The listing builds one solid part. Answer for the finished solid, in the listing's coordinates (mm). Face numbers are marked on the shaded views. Give positions to 0.01 mm unless a question says otherwise; leave off trailing zeros. Write each loop counter-clockwise with the first axis right and the second up, starting at its lowest first coordinate (ties: lowest second). Pieces come first, ordered by that corner, then holes. Notation, with made-up numbers: (36.25, 42.5) -> (94.25, 42.5) arc R21 cw to (94.25, 77.5) -> close; hole circle Ø7 at (35, -32.5). An arc over 180 degrees is marked (long way). Put each result on its own line as item: value. Start each with the question number.
1) A cutting plane is placed at D-D (z = -15). Write down the section's boundary in (x, y).
2) A cutting plane is placed at B-B (y = 3). Write down the section's boundary in (x, z), then the cut area to 3 significant figures.
3) Find the intervals of material crossed by line 1 along Z through (x, y) = (12.5, 5.5); line 2 along Y through (x, z) = (-4, -8.5); line 3 along Y through (x, z) = (0, -14), in increasing order. Write a range as from..to.
4) Flat-ended cylindrical pins translate along their axes: pin 1 Ø1.1 at (x, y) = (-21, 0.5) entering from +Z; pin 2 Ø0.5 at (x, y) = (22, 0.5) entering from -Z; pin 3 Ø4 at (x, y) = (-16, 3) entering from -Z; pin 4 Ø4 at (x, y) = (-7, 5) entering from +Z. Find the tip coordinate at first contact, or state that the pin passes through.
5) For a pull along Z with two mould halves and no side action, classify the marked faces 1, 2, 3 and 4 as released by +Z, released by -Z, zero draft, split by the parting line, or undercut.
6) A cutting plane is placed at C-C (x = -2.5). Write down the section's boundary in (y, z), then the cut area to 3 significant figures.
7) A cutting plane is placed at A-A (x = -20.5). Write down the section's boundary in (y, z), then the cut area to 3 significant figures.
from build123d import *

# Parameters (mm, degrees)
BOSS_EXTRUDE1_DEPTH   = 26.5
CUT_EXTRUDE1_DEPTH    = 2
MIRROR17_COPY_1_DEPTH = 26.5
MIRROR17_COPY_2_DEPTH = 2


with BuildPart() as part:
    # Sketch1 → Boss-Extrude1 (new body)
    with BuildSketch(Plane(origin=(0, 0, 0), x_dir=(0, 0, -1), z_dir=(1, 0, 0))):
        with BuildLine():
            Line((0, 0), (-12, 0))
            ThreePointArc((-12, 0), (-13.060660172, 0.439339828), (-13.5, 1.5))
            Line((-13.5, 1.5), (-13.5, 6))
            ThreePointArc((-13.5, 6), (-13.646446609, 6.353553391), (-14, 6.5))
            Line((-14, 6.5), (-17.5, 6.5))
            Line((-17.5, 6.5), (-17.5, 7.5))
            Line((-17.5, 7.5), (-14, 7.5))
            ThreePointArc((-14, 7.5), (-12.939339828, 7.060660172), (-12.5, 6))
            Line((-12.5, 6), (-12.5, 1.5))
            ThreePointArc((-12.5, 1.5), (-12.353553391, 1.146446609), (-12, 1))
            Line((-12, 1), (0, 1))
            Line((0, 1), (0, 0))
        make_face()
    boss_extrude1 = extrude(amount=BOSS_EXTRUDE1_DEPTH)

    # Sketch3 → Cut-Extrude1 (cut, through all)
    with BuildSketch(Plane(origin=(0, 1, 0), x_dir=(1, 0, 0), z_dir=(0, 1, 0))):
        with BuildLine():
            Line((26.5, 0), (16.5, 0))
            ThreePointArc((16.5, 0), (17.085786438, -1.414213562), (18.5, -2))
            Line((18.5, -2), (26.5, -2))
            Line((26.5, -2), (26.5, 0))
        make_face()
    cut_extrude1 = extrude(amount=-CUT_EXTRUDE1_DEPTH, mode=Mode.SUBTRACT)

    # Mirror16: Boss-Extrude1, Cut-Extrude1 across plane
    add(boss_extrude1.mirror(Plane(origin=(0, 0, 0), x_dir=(0, 0, 1), z_dir=(1, 0, 0))))
    add(cut_extrude1.mirror(Plane(origin=(0, 0, 0), x_dir=(0, 0, 1), z_dir=(1, 0, 0))), mode=Mode.SUBTRACT)

    # Mirror17: Boss-Extrude1, Cut-Extrude1 across plane
    add(boss_extrude1.mirror(Plane.XY))
    add(cut_extrude1.mirror(Plane.XY), mode=Mode.SUBTRACT)

    # Mirror17 copy 1 sketch → Mirror17 copy 1 (add)
    with BuildSketch(Plane.ZY):
        with BuildLine():
            Line((0, 0), (-12, 0))
            ThreePointArc((-12, 0), (-13.060660172, 0.439339828), (-13.5, 1.5))
            Line((-13.5, 1.5), (-13.5, 6))
            ThreePointArc((-13.5, 6), (-13.646446609, 6.353553391), (-14, 6.5))
            Line((-14, 6.5), (-17.5, 6.5))
            Line((-17.5, 6.5), (-17.5, 7.5))
            Line((-17.5, 7.5), (-14, 7.5))
            ThreePointArc((-14, 7.5), (-12.939339828, 7.060660172), (-12.5, 6))
            Line((-12.5, 6), (-12.5, 1.5))
            ThreePointArc((-12.5, 1.5), (-12.353553391, 1.146446609), (-12, 1))
            Line((-12, 1), (0, 1))
            Line((0, 1), (0, 0))
        make_face()
    extrude(amount=MIRROR17_COPY_1_DEPTH)

    # Mirror17 copy 2 sketch → Mirror17 copy 2 (cut, through all)
    with BuildSketch(Plane(origin=(0, 1, 0), x_dir=(-1, 0, 0), z_dir=(0, 1, 0))):
        with BuildLine():
            Line((26.5, 0), (16.5, 0))
            ThreePointArc((16.5, 0), (17.085786438, -1.414213562), (18.5, -2))
            Line((18.5, -2), (26.5, -2))
            Line((26.5, -2), (26.5, 0))
        make_face()
    extrude(amount=-MIRROR17_COPY_2_DEPTH, mode=Mode.SUBTRACT)


solid = part.part
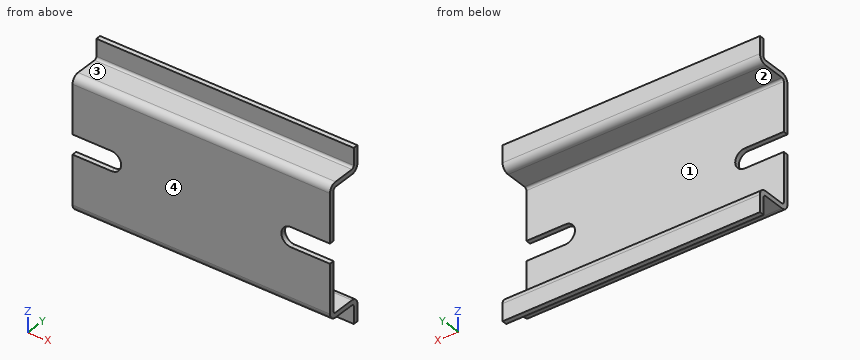
Reply:
1. outline: (-26.5, 6.5) -> (26.5, 6.5) -> (26.5, 7.5) -> (-26.5, 7.5) -> close
2. outline: (-26.5, -13.5) -> (26.5, -13.5) -> (26.5, -12.5) -> (-26.5, -12.5) -> close; (-26.5, 12.5) -> (26.5, 12.5) -> (26.5, 13.5) -> (-26.5, 13.5) -> close
2. area: 106 mm2
3. line 1: z = -13.5..-12.5, 12.5..13.5
3. line 2: y = 0..1
3. line 3: y = 6.5..7.5
4. pin 1: stops at z = 13.43
4. pin 2: stops at z = -13.3
4. pin 3: stops at z = -13.5
4. pin 4: stops at z = 17.5
5. face 1: undercut
5. face 2: undercut
5. face 3: released by +Z
5. face 4: zero draft
6. outline: (0, -12) arc R1.5 ccw to (1.5, -13.5) -> (6, -13.5) arc R0.5 cw to (6.5, -14) -> (6.5, -17.5) -> (7.5, -17.5) -> (7.5, -14) arc R1.5 ccw to (6, -12.5) -> (1.5, -12.5) arc R0.5 cw to (1, -12) -> (1, 12) arc R0.5 cw to (1.5, 12.5) -> (6, 12.5) arc R1.5 ccw to (7.5, 14) -> (7.5, 17.5) -> (6.5, 17.5) -> (6.5, 14) arc R0.5 cw to (6, 13.5) -> (1.5, 13.5) arc R1.5 ccw to (0, 12) -> close
6. area: 46.3 mm2
7. outline: (0, -12) arc R1.5 ccw to (1.5, -13.5) -> (6, -13.5) arc R0.5 cw to (6.5, -14) -> (6.5, -17.5) -> (7.5, -17.5) -> (7.5, -14) arc R1.5 ccw to (6, -12.5) -> (1.5, -12.5) arc R0.5 cw to (1, -12) -> (1, -2) -> (0, -2) -> close; (0, 2) -> (1, 2) -> (1, 12) arc R0.5 cw to (1.5, 12.5) -> (6, 12.5) arc R1.5 ccw to (7.5, 14) -> (7.5, 17.5) -> (6.5, 17.5) -> (6.5, 14) arc R0.5 cw to (6, 13.5) -> (1.5, 13.5) arc R1.5 ccw to (0, 12) -> close
7. area: 42.3 mm2
